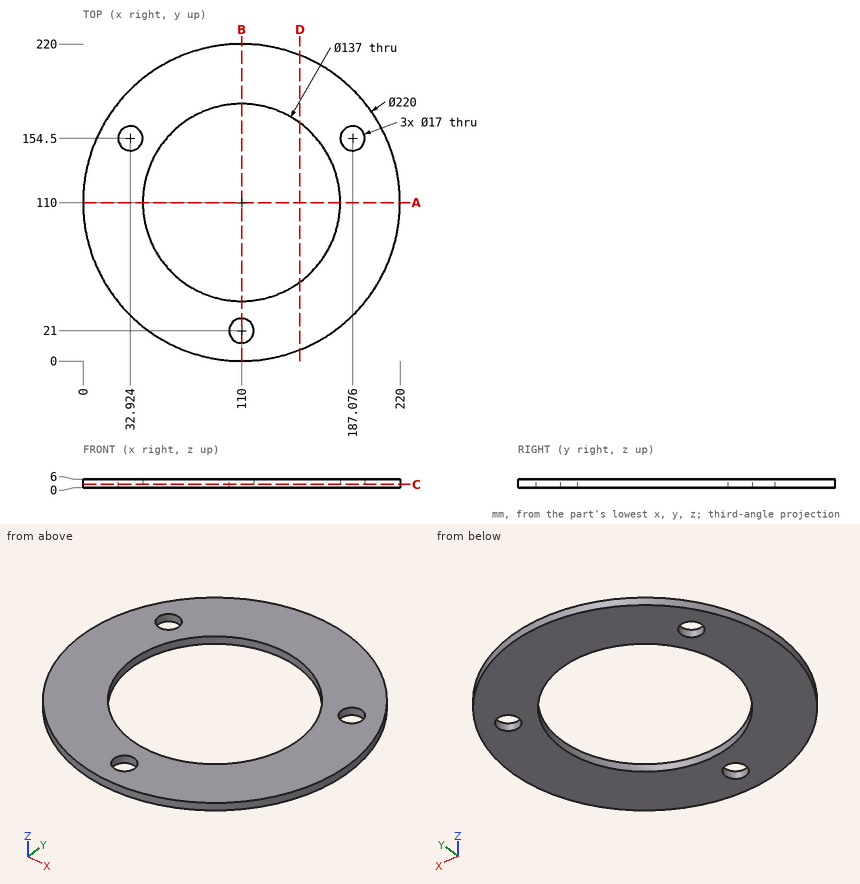
Design review of the part shown in the three views and the two pictorial views. Dimensions are in mm from the part's minimum x, y and z. Give positions to 0.01 mm unless a question says otherwise; leave off trailing zeros. Loops run counter-clockwise (first coordinate to the right, second up) from the corner with the lowest first, then second, coordinate; pieces in that order, holes last. Notation, with made-up numbers: M -35,-31.75 L 17,-31.75 A17 cw 17,-12.75 Z; hole C -20.5,-12.75 d10. An arc over 180 degrees is marked long. Answer as a JSON object with one key per item and string values. Group by question number.
Q1. For probe 1 along Y at (x, z) = (110, 2); probe 2 along Y at (x, z) = (111.5, 0.4); probe 3 along X at (y, z) = (67.5, 3.5), list the stretches that pass through material, from the lowest coordinate up. Write a range as [from, to].
Q2. Add section A-A on y = 110. Give the boundary of the cut face in (x, z).
Q3. Add section D-D on x = 150.5. Give the boundary of the cut face in (y, z) (1 decimal).
Q4. Add section C-C on z = 2.35. Give the boundary of the cut face in (x, y).
Q5. Add section B-B on x = 110. Give the boundary of the cut face in (y, z), and give its area (3 significant figures).
Q6. Insertion check: P1, Ø1.5, axis at y = 40, z = 2, coming from the -X side; P2, Ø3, axis at y = 178, z = 1.5, coming from the +X side; P3, Ø3, axis at y = 47.5, z = 1, coming from the +X side; P4, Ø13.5, axis at x = 32.92, y = 154.5, coming from the +Z side. Each pin has a flat end and moves straight along its axis. Give the tip position at first contact, or say it passes through.
Checked values:
{
 "1": {"probe 1": "[0, 12.5], [29.5, 41.5], [178.5, 220]", "probe 2": "[0.01, 12.63], [29.37, 41.52], [178.48, 219.99]", "probe 3": "[8.54, 56.28], [163.72, 211.46]"},
 "2": {"outline": "M 0,0 L 41.5,0 L 41.5,6 L 0,6 Z; M 178.5,0 L 220,0 L 220,6 L 178.5,6 Z"},
 "3": {"outline": "M 7.7,0 L 54.8,0 L 54.8,6 L 7.7,6 Z; M 165.2,0 L 212.3,0 L 212.3,6 L 165.2,6 Z"},
 "4": {"outline": "C 110,110 d220; hole C 32.92,154.5 d17; hole C 110,110 d137; hole C 110,21 d17; hole C 187.08,154.5 d17"},
 "5": {"outline": "M 0,0 L 12.5,0 L 12.5,6 L 0,6 Z; M 29.5,0 L 41.5,0 L 41.5,6 L 29.5,6 Z; M 178.5,0 L 220,0 L 220,6 L 178.5,6 Z", "area": "396 mm²"},
 "6": {"P1": "x = 24.53", "P2": "x = 197.62", "P3": "x = 201.54", "P4": "through"}
}
